Can you work these out from the drawing? Everything is in mm from the part's minimum corner. A direction names the side the tool comes from. Round coordinates to 2 decimals unless told otherwise and drop trailing zeros. Write each loop counter-clockwise with the first axis right and the second up, starting at its lowest first coordinate (ties: lowest second). Pieces come first, ordered by that corner, then holes. Notation, with made-up numbers: (39.5, -34) - (61.5, -34) arc R23 cw to (61.5, -1) - close; hole circle Ø11 at (-30, -27). An arc over 180 degrees is marked (long way). One line per item, written item: value. Start each with the question number.
(1) I'm going to push flat-ended pins straight in: pin 1 Ø9.5 at (x, z) = (75, 137.5) entering from -Y; pin 2 Ø12.5 at (x, z) = (138, 56.5) entering from +Y; pin 3 Ø1.5 at (y, z) = (5, 68.5) entering from -X; pin 4 Ø1.5 at (x, y) = (129, 13.5) entering from -Z. Where does each tip first touch, or does it pass through?
(2) If I drill on L1, parallel to Z at x = 68, y = 5.25; L2, parallel to Y at x = 21, z = 108; L3, parallel to X at y = 2, z = 33.5, over which ranges is the centre line in solid material (lowest first)? Write a range as from..to.
(3) On a 3-axis mill with a long thin cutter (end or side, diameter ignored), from which of +Z, -Z, +X, -X, +Y, -Y can I reach the whole of each face in a straight line? I mean the marked faces 3, 4, 5 and 6. Say none if no direction works.
(4) I want a section at D-D on x = 72.5. List the corners of the cut face in (y, z) for me.
(5) I want a section at A-A on y = 2.75. List the corners of the cut face in (x, z) for me.
(6) I want a section at B-B on z = 17. List the corners of the cut face in (x, y) for me, plus the area to 3 significant figures.
(7) I want a section at C-C on x = 99. List the corners of the cut face in (y, z) for me, plus the area to 3 significant figures.
(8) Thinking about a two-plate mould opening in Z: for the marked faces 1 and 2, which applies, +Z half, -Z half, draft (parallel to the pull), parting line (faces both ways), or undercut?
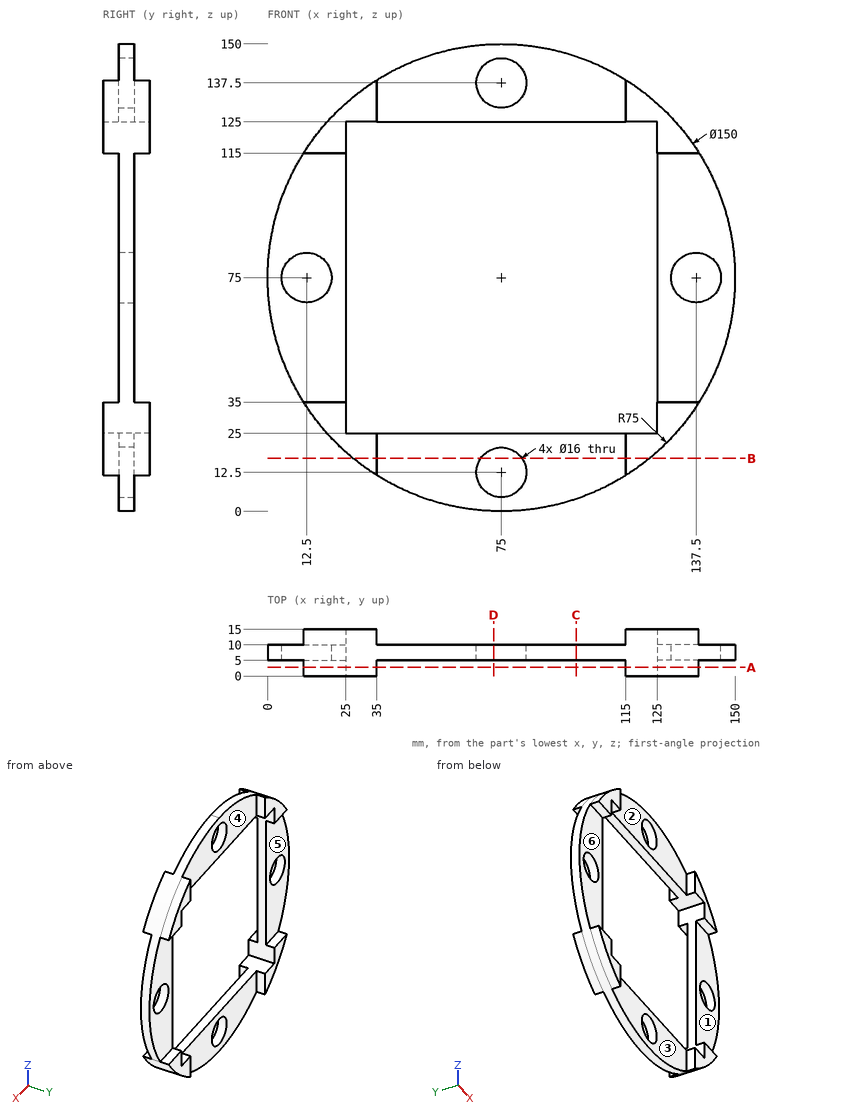
Established:
1. pin 1: through
1. pin 2: y = 10
1. pin 3: x = 0.22
1. pin 4: z = 22.18
2. L1: 0.33..8.63, 16.37..25, 125..133.63, 141.37..149.67
2. L2: 5..10
2. L3: 12.53..25, 125..137.47
3. face 3: +Z, -Z, -Y
3. face 4: +Z, -Z, +Y
3. face 5: +X, -X, +Y
3. face 6: +X, -X, -Y
4. outline: (5, 0.04) - (10, 0.04) - (10, 4.9) - (5, 4.9) - close; (5, 20.1) - (10, 20.1) - (10, 25) - (5, 25) - close; (5, 125) - (10, 125) - (10, 129.9) - (5, 129.9) - close; (5, 145.1) - (10, 145.1) - (10, 149.96) - (5, 149.96) - close
5. outline: (11.56, 35) arc R75 ccw to (35, 11.56) - (35, 25) - (25, 25) - (25, 35) - close; (11.56, 115) - (25, 115) - (25, 125) - (35, 125) - (35, 138.44) arc R75 ccw to start; (115, 11.56) arc R75 ccw to (138.44, 35) - (125, 35) - (125, 25) - (115, 25) - close; (115, 125) - (125, 125) - (125, 115) - (138.44, 115) arc R75 ccw to (115, 138.44) - close
6. outline: (27.45, 0) - (35, 0) - (35, 5) - (68.39, 5) - (68.39, 10) - (35, 10) - (35, 15) - (27.45, 15) - close; (81.61, 5) - (115, 5) - (115, 0) - (122.55, 0) - (122.55, 15) - (115, 15) - (115, 10) - (81.61, 10) - close
6. area: 560 mm2
7. outline: (5, 3.94) - (10, 3.94) - (10, 25) - (5, 25) - close; (5, 125) - (10, 125) - (10, 146.06) - (5, 146.06) - close
7. area: 211 mm2
8. face 1: undercut
8. face 2: draft
